Answer from the drawing. Dimensions are ordinates in mm from the lowest x, y and z of the part. Coordinates: 2 decimals unless noted, no trailing zeros. Write each loop counter-clockwise with the first axis right and the second up, starting at its lowest first coordinate (ties: lowest second). Pieces come first, ordered by that corner, then holes. Notation, with made-up numbers: (-19, -10) -> (-7, -10) arc R13 cw to (-7, -2) -> close; hole circle Ø10 at (82, -26.5). An arc over 180 degrees is marked (long way). One line per item, written item: value. Start each with the question number.
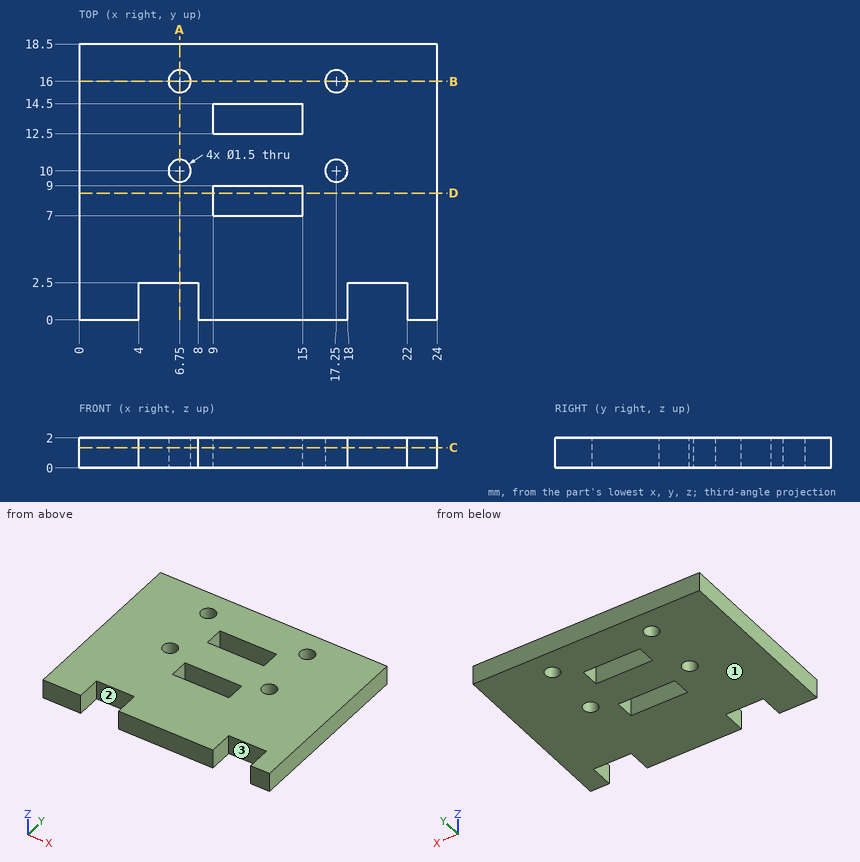
1. Given pin 1 (1.2 mm diameter, centred on x = 17.25, y = 10, fed in from -Z); pin 2 (1 mm diameter, centred on x = 6, z = 1, fed in from -Y), each flat-ended and moving along its own axis, determine where each tip first touches the part or whether it passes through.
2. A cutting plane is placed at B-B on y = 16. Give the vertices of the cut face in (x, z).
3. A cutting plane is placed at C-C on z = 1.35. Give the vertices of the cut face in (x, y), then the cut area to 3 significant figures.
4. A cutting plane is placed at A-A on x = 6.75. Give the vertices of the cut face in (y, z).
5. A cutting plane is placed at D-D on y = 8.5. Give the vertices of the cut face in (x, z), then the cut area to 3 significant figures.
6. Find the intervals of material crossed by probe 1 along Y at (x, z) = (10, 1.25); probe 2 along Y at (x, z) = (17.25, 1.15); probe 3 along X at (y, z) = (1.75, 1.6), in increasing order. Write a range as from..to.
7. For a pull along X with two mould halves and no side action, classify the marked faces 1, 2 and 3 as +X half, -X half, draft (parallel to the pull), parting line (faces both ways), or undercut.
Derived:
1. pin 1: passes through
1. pin 2: stops at y = 2.5
2. outline: (0, 0) -> (6, 0) -> (6, 2) -> (0, 2) -> close; (7.5, 0) -> (16.5, 0) -> (16.5, 2) -> (7.5, 2) -> close; (18, 0) -> (24, 0) -> (24, 2) -> (18, 2) -> close
3. outline: (0, 0) -> (4, 0) -> (4, 2.5) -> (8, 2.5) -> (8, 0) -> (18, 0) -> (18, 2.5) -> (22, 2.5) -> (22, 0) -> (24, 0) -> (24, 18.5) -> (0, 18.5) -> close; hole circle Ø1.5 at (6.75, 10); hole circle Ø1.5 at (6.75, 16); hole (9, 7) -> (15, 7) -> (15, 9) -> (9, 9) -> close; hole (9, 12.5) -> (15, 12.5) -> (15, 14.5) -> (9, 14.5) -> close; hole circle Ø1.5 at (17.25, 10); hole circle Ø1.5 at (17.25, 16)
3. area: 393 mm2
4. outline: (2.5, 0) -> (9.25, 0) -> (9.25, 2) -> (2.5, 2) -> close; (10.75, 0) -> (15.25, 0) -> (15.25, 2) -> (10.75, 2) -> close; (16.75, 0) -> (18.5, 0) -> (18.5, 2) -> (16.75, 2) -> close
5. outline: (0, 0) -> (9, 0) -> (9, 2) -> (0, 2) -> close; (15, 0) -> (24, 0) -> (24, 2) -> (15, 2) -> close
5. area: 36.0 mm2
6. probe 1: y = 0..7, 9..12.5, 14.5..18.5
6. probe 2: y = 0..9.25, 10.75..15.25, 16.75..18.5
6. probe 3: x = 0..4, 8..18, 22..24
7. face 1: draft
7. face 2: undercut
7. face 3: undercut
